Geometry check sheet. Reference: the model listing, model coordinates, mm. A direction names the side the tool comes from. Round coordinates to 2 decimals unless told otherwise and drop trailing zeros. Order: outer loops, then holes, each group sorted by start corner. A loop starts at its lowest first (then second) coordinate and runs counter-clockwise, first axis right, second up.
Autodesk Inventor part; units mm, degrees
ref_plane "YZ Plane" through (0, 0, 0) normal (1, 0, 0) x (0, 1, 0)
ref_plane "XZ Plane" through (0, 0, 0) normal (0, 1, 0) x (-1, 0, 0)
ref_plane "XY Plane" through (0, 0, 0) normal (0, 0, 1) x (1, 0, 0)
sketch "Sketch1" plane through (0, 0, 0) normal (1, 0, 0) x (0, 1, 0)
  line L0 (0, 8) -> (0, -8)
  line L1 (0, -8) -> (11, -8)
  line L2 (0, 8) -> (11, 8)
  line L3 (11, 8) -> (11, 13)
  line L4 (11, 13) -> (12.5, 13)
  line L5 (12.5, 13) -> (12.5, 8)
  line L6 (12.5, 8) -> (14.5, 8)
  line L7 (14.5, 8) -> (14.5, 15)
  line L8 (14.5, 15) -> (9, 15)
  line L9 (9, 15) -> (9, 10)
  line L10 (9, 10) -> (-3, 10)
  line L11 (-3, 10) -> (-4, 10)
  line L12 (-4, 10) -> (-4, 2.5)
  line L13 (0, 0) -> (3.5, 0)
  line L14 (0, -8) -> (11, -8)
  line L15 (11, -8) -> (11, -13)
  line L16 (11, -13) -> (12.5, -13)
  line L17 (12.5, -13) -> (12.5, -8)
  line L18 (14.5, -8) -> (14.5, -15)
  line L19 (14.5, -15) -> (9, -15)
  line L20 (9, -15) -> (9, -10)
  line L21 (9, -10) -> (-3, -10)
  line L22 (-3, -10) -> (-4, -10)
  line L23 (-4, -10) -> (-4, 2.5)
  line L24 (14.5, -8) -> (12.5, -8)
  point P0 (11.75, -15)
  point P1 (11.75, -13)
  dimension "d0" = 16
  dimension "d1" = 0
  dimension "d2" = 11
  dimension "d3" = 11
  dimension "d4" = 5
  dimension "d5" = 1.5
  dimension "d6" = 2
  dimension "d7" = 7
  dimension "d8" = 5.5
  dimension "d9" = 5
  dimension "d10" = 1
  dimension "d13" = 2
  dimension "d14" = 4
extrude "Extrusion1" add sketch "Sketch1" along normal blind 20
fillet "Fillet1" radius 5 2 edges at (10, 9, -10) (10, 9, 10)
chamfer "Chamfer1" distance 1 angle 45 12 edges at (20, 11, -10.5) (20, 11.75, -13) (20, 12.5, -10.5) (20, 11, 10.5) (20, 11.75, 13) (20, 12.5, 10.5) (0, 11, -10.5) (0, 11.75, -13) (0, 12.5, -10.5) (0, 11, 10.5) (0, 11.75, 13) (0, 12.5, 10.5)
sketch "Sketch2" plane through (0, 0, 8) normal (0, 1, 0) x (1, 0, 0)
  circle A0 centre (10, 7.5) radius 3
  line L0 (20, 16) -> (20, 0)
  line L1 (0, -7) -> (20, -7)
  line L2 (0, 0) -> (20, 0)
  point P0 (0, 8)
  dimension "d19" = 6
  dimension "d20" = 10
  dimension "d27" = 7.5
extrude "Extrusion2" cut sketch "Sketch2" against normal blind 20
chamfer "Chamfer2" distance 2.5 angle 45 1 edges at (7, 0, 0.5)
properties part number "Drziak_2"
(1) Sectioned sample at C-C, the plane y = 5. Record the cut outline in (x, z), and give its area (3 significant figures).
Returned:
outline: (0, -10.1) - (20, -10.1) - (20, -8) - (0, -8) - close; (0, 8) - (20, 8) - (20, 10.1) - (0, 10.1) - close
area: 84.0 mm2
(2) Depth check by flat-ended pin: P1, Ø1.5, axis at x = 2.5, y = 0.5, coming from the +Z side; P2, Ø6, axis at x = 14, y = 1.5, coming from the -Z side (3 decimals); P3, Ø9.5, axis at x = 10, z = 0.5, coming from the +Y side. Enter the tip coordinate at first touch or a pass-through.
Returned:
P1: stops at z = 10
P2: stops at z = -10.025
P3: stops at y = -0.75
(3) Set-up check for faces 4 (the flat face through (0.4, 11.7, -13.6)), 5 (the flat face through (19.5, 13, -11)), 6 (the flat face through (10, 12.5, -11)): record each of +Z, -Z, +X, -X, +Y, -Y from which the full face is reachable in a straight line by a thin tool's end or side.
Returned:
face 4: -X
face 5: +X
face 6: +X, -X
(4) Sectioned sample at A-A, the plane z = -9. Record the cut outline in (x, y).
Returned:
outline: (0, -4) - (20, -4) - (20, 10) - (19, 11) - (1, 11) - (0, 10) - close; (0, 13.5) - (1, 12.5) - (19, 12.5) - (20, 13.5) - (20, 14.5) - (0, 14.5) - close
(5) Material ranges on line 1 (Z direction, x = 10, y = -3.35); line 2 (X direction, y = -3.4, z = 0.5); line 3 (Z direction, x = 10.5, y = 2.5), recorded low to high.
Returned:
line 1: z = -10 to -2.5, 3.5 to 10
line 2: x = 0 to 7, 13 to 20
line 3: z = -10 to -8, 8 to 10
(6) Draft check along Y on faces 1 (the flat face through (10, 12, -13)), 2 (the flat face through (10, 5, 8)), 3 (the flat face through (9.9, 0, -5.2)). Enter one of: released by +Y, released by -Y, zero draft, split by the parting line, or undercut.
Returned:
face 1: undercut
face 2: zero draft
face 3: released by +Y
